Here's how the part is built. I have some questions about the finished solid (model axes, mm). Face numbers are marked on the shaded views. A direction names the side the tool comes from. Round coordinates to 2 decimals unless told otherwise and drop trailing zeros. Write each loop counter-clockwise with the first axis right and the second up, starting at its lowest first coordinate (ties: lowest second). Pieces come first, ordered by that corner, then holes. Notation, with made-up numbers: (83, 64.25) -> (100, 64.25) arc R21 cw to (100, 79.25) -> close; hole circle Ø4 at (38, 21). An arc over 180 degrees is marked (long way). Put each result on its own line as item: value. Start each with the question number.
1. I need wall thicknesses on probe 1 along X at (y, z) = (29.5, 0); probe 2 along Z at (x, y) = (0, 7). Which ranges of each line are inside material? Lowest first, please. Write a range as from..to.
2. Suppose I cut it at A-A (x = 0). Please give me the cut outline in (y, z), then the cut area to 3 significant figures.
3. Which directions (+Z, -Z, +X, -X, +Y, -Y) give clear straight access to the entire face, cutting with the end or side of a thin tool? Please do the marked faces 4 and 5.
4. We'd pull the mould along Z, two halves only. Please class the marked faces 1, 2 and 3: +Z half, -Z half, draft (parallel to the pull), parting line (faces both ways), or undercut.
5. Suppose I cut it at D-D (y = 28.5). Please give me the cut outline in (x, z).
6. For pin 1 (8 mm diameter, centred on x = 5, y = 15, fed in from -Z); pin 2 (1.5 mm diameter, centred on x = -1.5, y = 16.5, fed in from -Z); pin 3 (1.8 mm diameter, centred on x = 0, z = 1, fed in from -Y); pin 4 (6 mm diameter, centred on x = -4.5, z = -5, fed in from -Y), each with a flat end and sliding along its axis, tell me the tip position at first contact or that it passes through.
7. Suppose I cut it at B-B (y = 6.5). Please give me the cut outline in (x, z).
8. Suppose I cut it at C-C (y = 13). Please give me the cut outline in (x, z), then the cut area to 3 significant figures.
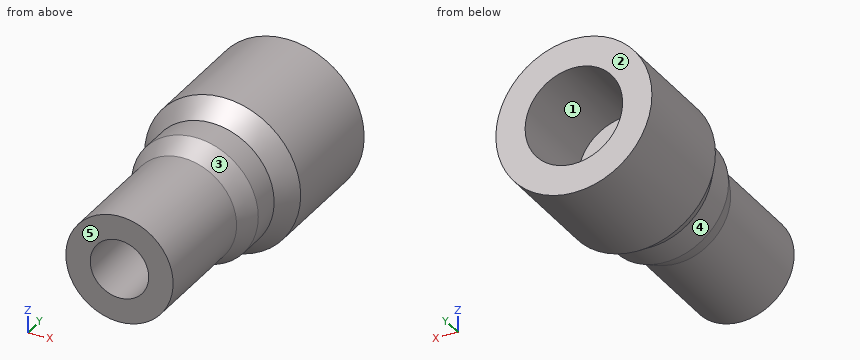
Autodesk Inventor part; units mm, degrees
ref_plane "Work Plane1" through (0, 14.25, 0) normal (0, 1, 0) x (1, 0, 0)
ref_plane "Work Plane2" through (0, 19.5, 0) normal (0, 1, 0) x (1, 0, 0)
ref_plane "YZ Plane" through (0, 0, 0) normal (1, 0, 0) x (0, 1, 0)
sketch "Sketch1" plane through (0, 0, 0) normal (0, 1, 0) x (-1, 0, 0)
  circle A0 centre (0, 0) radius 5.5
  dimension "d0" = 11
extrude "Extrusion1" add sketch "Sketch1" along normal blind 12
sketch "Sketch2" plane through (0, 0, 0) normal (0, -1, 0) x (1, 0, 0)
  circle A0 centre (0, 0) radius 3
  dimension "d3" = 6
extrude "Extrusion2" cut sketch "Sketch2" against normal blind 10
ref_plane "Work Plane1" through (0, 14.25, 0) normal (0, 1, 0) x (1, 0, 0)
sketch "Sketch3" plane through (0, 14.25, 0) normal (0, 1, 0) x (1, 0, 0)
  circle A0 centre (0, 0) radius 5.5
  circle A1 centre (0, 0) radius 6.5
  dimension "d7" = 13
extrude "Extrusion3" add sketch "Sketch3" along normal blind 3 contours A0 | A1
loft "Loft1" add section 1 edges at (5.5, 12, 0) section 2 edges at (-6.5, 14.25, 0)
ref_plane "Work Plane2" through (0, 19.5, 0) normal (0, 1, 0) x (1, 0, 0)
sketch "Sketch4" plane through (0, 19.5, 0) normal (0, 1, 0) x (1, 0, 0)
  circle A0 centre (0, 0) radius 3
  circle A1 centre (0, 0) radius 8
  dimension "d15" = 16
extrude "Extrusion4" add sketch "Sketch4" along normal blind 12 contours A0 | A1
loft "Loft2" add section 1 edges at (-6.5, 17.25, 0) section 2 edges at (-8, 19.5, 0)
sketch "Sketch5" plane through (0, 31.5, 0) normal (0, 1, 0) x (1, 0, 0)
  circle A0 centre (0, 0) radius 8
  circle A1 centre (0, 0) radius 5
  dimension "d22" = 10
extrude "Extrusion5" cut sketch "Sketch5" against normal blind 10 contours A1
properties part number "reductor_10_6"
Verdict:
1. probe 1: x = -8..-5, 5..8
1. probe 2: z = -5.5..-3, 3..5.5
2. outline: (0, -5.5) -> (12, -5.5) -> (14.25, -6.5) -> (17.25, -6.5) -> (19.5, -8) -> (31.5, -8) -> (31.5, -5) -> (21.5, -5) -> (21.5, 5) -> (31.5, 5) -> (31.5, 8) -> (19.5, 8) -> (17.25, 6.5) -> (14.25, 6.5) -> (12, 5.5) -> (0, 5.5) -> (0, 3) -> (10, 3) -> (10, -3) -> (0, -3) -> close
2. area: 263 mm^2
3. face 4: -Y
3. face 5: +Z, -Z, +X, -X, -Y
4. face 1: undercut
4. face 2: draft
4. face 3: parting line
5. outline: circle Ø16 at (0, 0); hole circle Ø10 at (0, 0)
6. pin 1: stops at z = -6.67
6. pin 2: stops at z = -6.46
6. pin 3: stops at y = 10
6. pin 4: stops at y = 0
7. outline: circle Ø11 at (0, 0); hole circle Ø6 at (0, 0)
8. outline: circle Ø11.89 at (0, 0)
8. area: 111 mm^2
